Geometry check sheet. Reference: the model listing, model coordinates, mm. Face numbers are marked on the shaded views. A direction names the side the tool comes from. Coordinates: 2 decimals unless noted, no trailing zeros. Loops run counter-clockwise (first coordinate to the right, second up) from the corner with the lowest first, then second, coordinate; pieces in that order, holes last. Notation, with made-up numbers: (78, -11.75) - (111, -11.75) arc R30 cw to (111, 12.25) - close; hole circle Ø8 at (49, 49.5). An arc over 180 degrees is marked (long way). Write each question's results on one line, items separated by ' | '. Start each with the question number.
(1) Sectioned sample at D-D (z = 13.5). Enter the section's corners in (x, y).
(2) Sectioned sample at C-C (z = 0). Enter the section's corners in (x, y), plus the area to 3 significant figures.
(3) Go/stop test with flat-tipped pins: pin 1 Ø2.5 at (x, y) = (55, 6.5) entering from +Z; pin 2 Ø8 at (y, z) = (37.5, -1.5) entering from -X; pin 3 Ø12 at (x, z) = (26.5, 2) entering from +Y. Record where each tip stops, or that it passes through.
(4) Sectioned sample at B-B (x = 20). Enter the section's corners in (y, z).
(5) Mould release check, pull along Z, two halves, no side actions. Record for the marked faces 5, 6, 7 and 8: pulls with the +Z half, pulls with the -Z half, needs draft (parallel to the pull), parting line crosses it, or undercut.
(6) Access from +Z, -Z, +X, -X, +Y, -Y to the whole of each face (thin tool, end or side, straight path). Record for the marked faces 1, 2, 3 and 4.
(7) Sectioned sample at A-A (y = 105). Enter the section's corners in (x, z), plus the area to 3 significant figures.
(8) Material ranges on probe 1 along X at (y, z) = (19, -14); probe 2 along Y at (x, z) = (59.4, 1); probe 3 along Y at (x, z) = (41.5, -2), recorded low to high.
from build123d import *

# Parameters (mm, degrees)
SALIENTE_EXTRUIR1_DEPTH      = 3
SALIENTE_EXTRUIR1_2_DEPTH    = 3
SALIENTE_EXTRUIR2_DEPTH      = 3
SALIENTE_EXTRUIR2_DEPTH_BACK = 3
CROQUIS4_W                   = 4
CROQUIS4_H                   = 30
SALIENTE_EXTRUIR3_DEPTH      = 110
SALIENTE_EXTRUIR4_DEPTH      = 56
CORTAR_EXTRUIR1_DEPTH        = 4
CROQUIS7_R                   = 5
CORTAR_EXTRUIR2_DEPTH        = 4


with BuildPart() as part:
    # Croquis2 → Saliente-Extruir1 (new body)
    with BuildSketch(Plane(origin=(0, 0, 0), x_dir=(1, 0, 0), z_dir=(0, 1, 0))):
        with BuildLine():
            Line((-5.5, -17.5), (5.5, -17.5))
            ThreePointArc((5.5, -17.5), (6.914213562, -16.914213562), (7.5, -15.5))
            Line((7.5, -15.5), (7.5, 15.5))
            ThreePointArc((7.5, 15.5), (6.914213562, 16.914213562), (5.5, 17.5))
            Line((5.5, 17.5), (-5.5, 17.5))
            ThreePointArc((-5.5, 17.5), (-6.914213562, 16.914213562), (-7.5, 15.5))
            Line((-7.5, 15.5), (-7.5, -15.5))
            ThreePointArc((-7.5, -15.5), (-6.914213562, -16.914213562), (-5.5, -17.5))
        make_face()
    extrude(amount=SALIENTE_EXTRUIR1_DEPTH)



with BuildPart() as body_2:
    # Croquis2 → Saliente-Extruir1 2 (new body)
    with BuildSketch(Plane(origin=(0, 0, 0), x_dir=(1, 0, 0), z_dir=(0, 1, 0))):
        with BuildLine():
            Line((52.5, -15.5), (52.5, 15.5))
            ThreePointArc((52.5, 15.5), (53.085786438, 16.914213562), (54.5, 17.5))
            Line((54.5, 17.5), (65.5, 17.5))
            ThreePointArc((65.5, 17.5), (66.914213562, 16.914213562), (67.5, 15.5))
            Line((67.5, 15.5), (67.5, -15.5))
            ThreePointArc((67.5, -15.5), (66.914213562, -16.914213562), (65.5, -17.5))
            Line((65.5, -17.5), (54.5, -17.5))
            ThreePointArc((54.5, -17.5), (53.085786438, -16.914213562), (52.5, -15.5))
        make_face()
    extrude(amount=SALIENTE_EXTRUIR1_2_DEPTH)


with BuildPart() as part_1:
    add(part.part)

    add(body_2.part)  # Saliente-Extruir2 merges body 2
    # Croquis3 → Saliente-Extruir2 (add, two sides: drawn at the far end of the back side and taken through both)
    with BuildSketch(Plane.XY.offset(-SALIENTE_EXTRUIR2_DEPTH_BACK)):
        Polygon((-7.5, 3), (-2, 8), (-2, 3), align=None)
        Polygon((2, 3), (7.5, 3), (2, 8), align=None)
        Polygon((52.5, 3), (58, 8), (58, 3), align=None)
        Polygon((62, 3), (67.5, 3), (62, 8), align=None)
    extrude(amount=SALIENTE_EXTRUIR2_DEPTH + SALIENTE_EXTRUIR2_DEPTH_BACK)

    # Croquis4 → Saliente-Extruir3 (add)
    with BuildSketch(Plane(origin=(0, 3, 0), x_dir=(1, 0, 0), z_dir=(0, 1, 0))):
        Rectangle(CROQUIS4_W, CROQUIS4_H)
        with Locations((60, 0)):
            Rectangle(CROQUIS4_W, CROQUIS4_H)
    extrude(amount=SALIENTE_EXTRUIR3_DEPTH)

    # Croquis5 → Saliente-Extruir4 (add)
    with BuildSketch(Plane(origin=(2, 0, 0), x_dir=(0, 0, -1), z_dir=(1, 0, 0))):
        Polygon((-15, 113), (-11.8, 113), (-11.8, 89), (11.8, 89), (11.8, 113), (15, 113), (15, 83), (11.5, 83), (-11.5, 83), (-15, 83), align=None)
    extrude(amount=SALIENTE_EXTRUIR4_DEPTH)

    # Croquis6 → Cortar-Extruir1 (cut)
    with BuildSketch(Plane.ZY.offset(2)):
        with BuildLine():
            Line((-9.55, 101), (-9.55, 113))
            Line((-9.55, 113), (9.55, 113))
            Line((9.55, 113), (9.55, 101))
            ThreePointArc((9.55, 101), (0, 91.45), (-9.55, 101))
        make_face()
    extrude(amount=-CORTAR_EXTRUIR1_DEPTH, mode=Mode.SUBTRACT)

    # Croquis7 → Cortar-Extruir2 (cut)
    with BuildSketch(Plane(origin=(62, 0, 0), x_dir=(0, 0, -1), z_dir=(1, 0, 0))):
        with Locations((-1, 105)):
            Circle(CROQUIS7_R)
    extrude(amount=-CORTAR_EXTRUIR2_DEPTH, mode=Mode.SUBTRACT)


solid = part_1.part
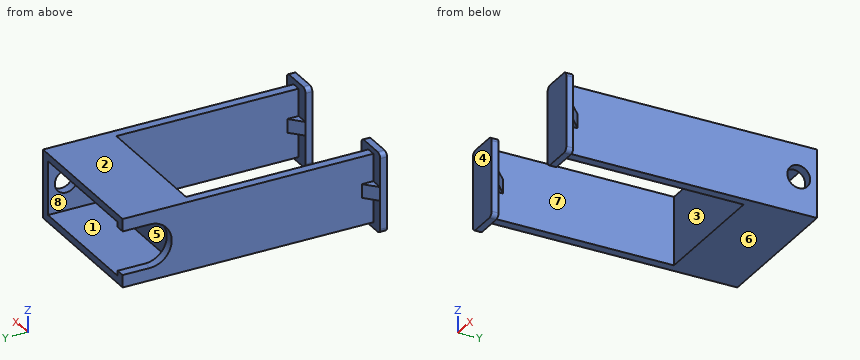
Outcome:
1) outline: (-7.5, 0) - (7.5, 0) - (7.5, 3) - (2, 3) - (2, 83) - (58, 83) - (58, 3) - (52.5, 3) - (52.5, 0) - (67.5, 0) - (67.5, 3) - (62, 3) - (62, 113) - (-2, 113) - (-2, 3) - (-7.5, 3) - close
2) outline: (-7.5, 0) - (7.5, 0) - (7.5, 3) - (2, 8) - (2, 83) - (58, 83) - (58, 8) - (52.5, 3) - (52.5, 0) - (67.5, 0) - (67.5, 3) - (62, 8) - (62, 100.1) - (58, 100.1) - (58, 89) - (2, 89) - (2, 91.45) - (-2, 91.45) - (-2, 8) - (-7.5, 3) - close; (58, 109.9) - (62, 109.9) - (62, 113) - (58, 113) - close | area: 1,240 mm2
3) pin 1: stops at z = 3 | pin 2: stops at x = -2 | pin 3: stops at y = 89
4) outline: (83, -15) - (113, -15) - (113, -11.8) - (89, -11.8) - (89, 11.8) - (113, 11.8) - (113, 15) - (83, 15) - close
5) face 5: undercut | face 6: pulls with the -Z half | face 7: needs draft | face 8: undercut
6) face 1: +Y | face 2: +Z, +X, -X, +Y | face 3: +Z, -Z | face 4: +Z, -Z, +X, -X, -Y
7) outline: (-2, -15) - (62, -15) - (62, -4) - (58, -4) - (58, -11.8) - (2, -11.8) - (2, -9.55) - (-2, -9.55) - close; (-2, 9.55) - (2, 9.55) - (2, 11.8) - (58, 11.8) - (58, 6) - (62, 6) - (62, 15) - (-2, 15) - close | area: 482 mm2
8) probe 1: x = -2 to 2, 58 to 62 | probe 2: y = 0 to 100, 110 to 113 | probe 3: y = 83 to 89
